Here's how the part is built. I have some questions about the finished solid (model axes, mm). Give positions to 0.01 mm unless a question says otherwise; leave off trailing zeros. Write each loop counter-clockwise with the first axis right and the second up, starting at its lowest first coordinate (ties: lowest second). Pieces come first, ordered by that corner, then holes. Notation, with made-up numbers: (61, -12.5) -> (79, -12.5) arc R10 ccw to (79, 6.5) -> close; hole circle Ø1 at (-37, 46.5). An arc over 180 degrees is marked (long way). Return JSON: item names as keys, results as strings.
from build123d import *

# Parameters (mm, degrees)
F0_R     = 17.5
F1_DEPTH = 25
F2_T     = -2
F3_R     = 3
F4_DEPTH = 19.6


with BuildPart() as f1:
    # F0 (on Top) → F1 (new body)
    with BuildSketch(Plane.XY):
        Circle(F0_R)
    extrude(amount=F1_DEPTH)

    # F2
    f2_openings = [f1.faces().sort_by_distance(p)[0] for p in [
        (0, 0, 0),
    ]]
    offset(amount=F2_T, openings=f2_openings)

    # F3 (on Front) → F4 (cut, symmetric)
    with BuildSketch(Plane.XZ):
        with Locations((0, 8)):
            Circle(F3_R)
    extrude(amount=F4_DEPTH, both=True, mode=Mode.SUBTRACT)


solid = f1.part
1. Suppose I cut it at B-B, the plane z = 8. List the corners of the cut face in (x, y) for me, and give its area (3 significant figures).
Taken from the geometry:
{"outline": "(-3, -17.24) -> (-3, -15.21) arc R15.5 cw to (-3, 15.21) -> (-3, 17.24) arc R17.5 ccw to start; (3, -17.24) arc R17.5 ccw to (3, 17.24) -> (3, 15.21) arc R15.5 cw to (3, -15.21) -> close", "area": "183 mm²"}
2. If I drill on line 1 (Z direction, x = 0, y = -16.8); line 2 (X direction, y = -0.5, z = 11.75); line 3 (Y direction, x = 0, z = 17.5), over which ranges is the centre line in solid material (lowest first)? Write a range as [from, to].
Taken from the geometry:
{"line 1": "z = [0, 5], [11, 25]", "line 2": "x = [-17.49, -15.49], [15.49, 17.49]", "line 3": "y = [-17.5, -15.5], [15.5, 17.5]"}
3. Suppose I cut it at D-D, the plane x = 11.5. List the corners of the cut face in (y, z) for me.
Taken from the geometry:
{"outline": "(-13.19, 0) -> (-10.39, 0) -> (-10.39, 23) -> (10.39, 23) -> (10.39, 0) -> (13.19, 0) -> (13.19, 25) -> (-13.19, 25) -> close"}
4. Suppose I cut it at A-A, the plane x = 0. List the corners of the cut face in (y, z) for me.
Taken from the geometry:
{"outline": "(-17.5, 0) -> (-15.5, 0) -> (-15.5, 5) -> (-17.5, 5) -> close; (-17.5, 11) -> (-15.5, 11) -> (-15.5, 23) -> (15.5, 23) -> (15.5, 11) -> (17.5, 11) -> (17.5, 25) -> (-17.5, 25) -> close; (15.5, 0) -> (17.5, 0) -> (17.5, 5) -> (15.5, 5) -> close"}
5. Suppose I cut it at C-C, the plane y = 0. List the corners of the cut face in (x, z) for me.
Taken from the geometry:
{"outline": "(-17.5, 0) -> (-15.5, 0) -> (-15.5, 23) -> (15.5, 23) -> (15.5, 0) -> (17.5, 0) -> (17.5, 25) -> (-17.5, 25) -> close"}
6. For pin 1 Ø9.5 at (x, y) = (1, 1) entering from -Z; pin 2 Ø1 at (x, z) = (8, 16.5) entering from +Y; pin 3 Ø4 at (x, z) = (-7, 9) entering from -Y, each with a flat end and sliding along its axis, tell me the tip position at first contact or that it passes through.
Taken from the geometry:
{"pin 1": "stops at z = 23", "pin 2": "stops at y = 15.81", "pin 3": "stops at y = -16.77"}
7. If we mould it in two halves opening along Y, with no side actions, what happens to faces 1 (the face through (-3.36, -15.13, 11.34)), 2 (the face through (0, 0, 23)), 3 (the face through (0, 0, 25)), 4 (the face through (-3.794, -17.084, 12.325))? For each: released by +Y, released by -Y, zero draft, split by the parting line, or undercut.
Taken from the geometry:
{"face 1": "undercut", "face 2": "undercut", "face 3": "zero draft", "face 4": "split by the parting line"}
